Model file for the job. Use its own axes, mm. A direction names the side the tool comes from. Round coordinates to 2 decimals unless told otherwise and drop trailing zeros. Order: outer loops, then holes, each group sorted by start corner. A loop starts at its lowest first (then second) coordinate and runs counter-clockwise, first axis right, second up. Notation, with made-up numbers: M -37,54.25 L 1,54.25 A24 ccw 1,72.25 Z; hole C 12.5,-10 d7. An arc over 180 degrees is marked long. Return JSON: item names as keys, results as strings. Group by question number.
Item 1: Pull direction X, two halves, no side cores. Call faces 1 (the face through (0, 4, -4.5)), 2 (the face through (-12.2, 3, 4)), 3 (the face through (5.98, 3.01, -1.02)): pulls with the +X half, pulls with the -X half, needs draft (parallel to the pull), parting line crosses it, or undercut.
Item 2: Slice it at D-D on y = 5. Write the cut outline in (x, z), then the cut area to 3 significant figures.
Item 3: Pin check, flat tips, straight feed: pin 1 Ø1.8 at (y, z) = (3, 5.5) entering from -X; pin 2 Ø2 at (x, y) = (-6.2, 3) entering from +Z; pin 3 Ø1.8 at (x, y) = (-14, 3.5) entering from +Z. Stop position of each tip, or through.
Item 4: Slice it at A-A on y = 0.75. Write the cut outline in (x, z).
Item 5: Which spindle directions (+Z, -Z, +X, -X, +Y, -Y) get a long thin tool onto all of the face, cutting with end or side? Do faces 4 (the face through (0, 6, 2)), 5 (the face through (-15, 3, 0)), 6 (the face through (15, 3, 0)), 7 (the face through (7.121, 3.845, 3.791)). Say none if no direction does.
Item 6: Probe line 1 along X through (y, z) = (3, 4.75); line 2 along Y through (x, z) = (-6.2, 5.75); line 3 along Z through (x, y) = (-15, 3). List the from-to ranges inside material, lowest first.
Item 7: Slice it at B-B on z = 7. Write the cut outline in (x, y), then the cut area to 3 significant figures.
Item 8: Slice it at C-C on x = -10.5. Write the cut outline in (y, z).
from build123d import *

# Parameters (mm, degrees)
ESBO_O1_W                     = 24.4
ESBO_O1_H                     = 6
RESSALTO_EXTRUS_O1_DEPTH      = 8.1
ESBO_O3_W                     = 36.4
ESBO_O3_H                     = 6
RESSALTO_EXTRUS_O2_DEPTH      = 4.5
CHANFRO1_SIZE                 = 2
FURO_ROSCADO_DE_M3X0_51_D     = 2.5
FURO_ROSCADO_DE_M3X0_51_DEPTH = 8.5
FURO_ROSCADO_DE_M3X0_51_TIP   = 0.751075774


with BuildPart() as part:
    # Esboço1 → Ressalto-extrusão1 (new body)
    with BuildSketch(Plane.XY):
        with Locations((0, 3)):
            Rectangle(ESBO_O1_W, ESBO_O1_H)
    extrude(amount=RESSALTO_EXTRUS_O1_DEPTH)

    # Esboço3 → Ressalto-extrusão2 (add)
    with BuildSketch(Plane(origin=(0, 0, 0), x_dir=(-1, 0, 0), z_dir=(0, 0, -1))):
        with Locations((0, 3)):
            Rectangle(ESBO_O3_W, ESBO_O3_H)
    extrude(amount=RESSALTO_EXTRUS_O2_DEPTH)

    # Chanfro1
    chanfro1_edges = [part.edges().sort_by_distance(p)[0] for p in [
        (0, 0, -4.5),
    ]]
    chamfer(chanfro1_edges, length=CHANFRO1_SIZE)

    # Furo roscado de M3x0.51
    with Locations(Plane.XY.offset(8.1)):
        with Locations((-6.2, 3), (6.2, 3)):
            Hole(FURO_ROSCADO_DE_M3X0_51_D / 2, depth=FURO_ROSCADO_DE_M3X0_51_DEPTH)
            with Locations((0, 0, -(FURO_ROSCADO_DE_M3X0_51_DEPTH + FURO_ROSCADO_DE_M3X0_51_TIP / 2))):  # 118° drill point
                Cone(0, FURO_ROSCADO_DE_M3X0_51_D / 2, FURO_ROSCADO_DE_M3X0_51_TIP, mode=Mode.SUBTRACT)


solid = part.part
Output values:
{
 "1": {"face 1": "needs draft", "face 2": "pulls with the -X half", "face 3": "undercut"},
 "2": {"outline": "M -18.2,-4.5 L 18.2,-4.5 L 18.2,0 L 12.2,0 L 12.2,8.1 L -12.2,8.1 L -12.2,0 L -18.2,0 Z", "area": "361 mm²"},
 "3": {"pin 1": "x = -12.2", "pin 2": "z = -0.55", "pin 3": "z = 0"},
 "4": {"outline": "M -18.2,-3.25 L 18.2,-3.25 L 18.2,0 L 12.2,0 L 12.2,8.1 L -12.2,8.1 L -12.2,0 L -18.2,0 Z"},
 "5": {"face 4": "+Z, -Z, +X, -X, +Y", "face 5": "+Z, -X, +Y, -Y", "face 6": "+Z, +X, +Y, -Y", "face 7": "+Z"},
 "6": {"line 1": "-12.2 to -7.45, -4.95 to 4.95, 7.45 to 12.2", "line 2": "0 to 1.75, 4.25 to 6", "line 3": "-4.5 to 0"},
 "7": {"outline": "M -12.2,0 L 12.2,0 L 12.2,6 L -12.2,6 Z; hole C -6.2,3 d2.5; hole C 6.2,3 d2.5", "area": "137 mm²"},
 "8": {"outline": "M 0,-2.5 L 2,-4.5 L 6,-4.5 L 6,8.1 L 0,8.1 Z"}
}
